Part model, mm, in its own coordinate system. A direction names the side the tool comes from. Round coordinates to 2 decimals unless told otherwise and drop trailing zeros. Loops run counter-clockwise (first coordinate to the right, second up) from the corner with the lowest first, then second, coordinate; pieces in that order, holes last. Notation, with made-up numbers: (75.25, 70) -> (125.25, 70) arc R34 cw to (125.25, 102) -> close; hole circle Ø5 at (78.5, 32). An arc over 180 degrees is marked (long way). Answer as a JSON object with one key per item and string values. Group by question number.
from build123d import *

# Parameters (mm, degrees)
F0_R     = 2.25
F1_DEPTH = 4
F2_R     = 2.05
F3_DEPTH = 5
F4_W     = 13
F4_H     = 11
F5_DEPTH = 1


with BuildPart() as f1:
    # F0 (on Top) → F1 (new body)
    with BuildSketch(Plane.XY):
        with BuildLine():
            ThreePointArc((40, 5.119438), (39.414214, 6.533651), (38, 7.119438))
            Line((38, 7.119438), (-38, 7.119438))
            ThreePointArc((-38, 7.119438), (-39.414214, 6.533651), (-40, 5.119438))
            Line((-40, 5.119438), (-40, -5.119438))
            ThreePointArc((-40, -5.119438), (-39.414214, -6.533651), (-38, -7.119438))
            Line((-38, -7.119438), (38, -7.119438))
            ThreePointArc((38, -7.119438), (39.414214, -6.533651), (40, -5.119438))
            Line((40, -5.119438), (40, 5.119438))
        make_face()
        with Locations((-35, 0)):
            Circle(F0_R, mode=Mode.SUBTRACT)
        with Locations((35, 0)):
            Circle(F0_R, mode=Mode.SUBTRACT)
    extrude(amount=F1_DEPTH)

    # F2 (on face) → F3 (cut)
    with BuildSketch(Plane.XY.offset(4)):
        with Locations((-15.9661, 0)):
            Circle(F2_R)
    extrude(amount=-F3_DEPTH, mode=Mode.SUBTRACT)

    # F4 (on face) → F5 (cut)
    with BuildSketch(Plane.XY.offset(4)):
        with Locations((-15.9661, 0)):
            Rectangle(F4_W, F4_H)
    extrude(amount=-F5_DEPTH, mode=Mode.SUBTRACT)


solid = f1.part
Item 1: Band-saw the part on C-C, the plane z = 0.65. List the corners of the cut face in (x, y), plus the area to 3 significant figures.
Item 2: Band-saw the part on A-A, the plane y = 0. List the corners of the cut face in (x, z).
Item 3: Drill centre lines: line 1 (Y direction, x = -16, z = 1.4); line 2 (Y direction, x = -35, z = 3.25); line 3 (X direction, y = -1, z = 0.35). Where is each one in solid material? Low to high.
Item 4: Drop flat-ended pins along their axis: pin 1 Ø4 at (x, y) = (-35, 0) entering from -Z; pin 2 Ø1.5 at (x, y) = (18.5, -1) entering from -Z. Give the stop position or say it passes through.
Item 5: Two-plate mould, pull along Y, no slides. Class faces 1 (the face through (37.08, -0.86, 1.97)), 2 (the face through (-32.92, -0.86, 1.97)), 3 (the face through (1, 7.119, 2)), 4 (the face through (-1, 0, 0)): pulls with the +Y half, pulls with the -Y half, needs draft (parallel to the pull), parting line crosses it, or undercut.
Item 6: Which spindle directions (+Z, -Z, +X, -X, +Y, -Y) get a long thin tool onto all of the face, cutting with end or side? Do faces 5 (the face through (-40, 0, 2)), 6 (the face through (-16, 3, 3)). Say none if no direction does.
Item 7: Band-saw the part on B-B, the plane x = -35. List the corners of the cut face in (y, z), plus the area to 3 significant figures.
Item 8: Band-saw the part on D-D, the plane y = -4.25. List the corners of the cut face in (x, z), plus the area to 3 significant figures.
Entries:
{
 "1": {"outline": "(-40, -5.12) arc R2 ccw to (-38, -7.12) -> (38, -7.12) arc R2 ccw to (40, -5.12) -> (40, 5.12) arc R2 ccw to (38, 7.12) -> (-38, 7.12) arc R2 ccw to (-40, 5.12) -> close; hole circle Ø4.5 at (-35, 0); hole circle Ø4.1 at (-15.97, 0); hole circle Ø4.5 at (35, 0)", "area": "1,090 mm²"},
 "2": {"outline": "(-40, 0) -> (-37.25, 0) -> (-37.25, 4) -> (-40, 4) -> close; (-32.75, 0) -> (-18.02, 0) -> (-18.02, 3) -> (-22.47, 3) -> (-22.47, 4) -> (-32.75, 4) -> close; (-13.92, 0) -> (32.75, 0) -> (32.75, 4) -> (-9.47, 4) -> (-9.47, 3) -> (-13.92, 3) -> close; (37.25, 0) -> (40, 0) -> (40, 4) -> (37.25, 4) -> close"},
 "3": {"line 1": "-7.12 to -2.05, 2.05 to 7.12", "line 2": "-7.12 to -2.25, 2.25 to 7.12", "line 3": "-40 to -37.02, -32.98 to -17.76, -14.18 to 32.98, 37.02 to 40"},
 "4": {"pin 1": "through", "pin 2": "z = 0"},
 "5": {"face 1": "undercut", "face 2": "undercut", "face 3": "pulls with the +Y half", "face 4": "needs draft"},
 "6": {"face 5": "+Z, -Z, -X, +Y, -Y", "face 6": "+Z"},
 "7": {"outline": "(-7.12, 0) -> (-2.25, 0) -> (-2.25, 4) -> (-7.12, 4) -> close; (2.25, 0) -> (7.12, 0) -> (7.12, 4) -> (2.25, 4) -> close", "area": "39.0 mm²"},
 "8": {"outline": "(-40, 0) -> (40, 0) -> (40, 4) -> (-9.47, 4) -> (-9.47, 3) -> (-22.47, 3) -> (-22.47, 4) -> (-40, 4) -> close", "area": "307 mm²"}
}
